Autodesk Inventor part; units mm, degrees
ref_plane "作業平面1" through (0, 0, 1.5) normal (0, 0, 1) x (1, 0, 0)
ref_plane "作業平面2" through (0, 0, 0.1) normal (0, 0, 1) x (1, 0, 0)
ref_plane "YZ Plane" through (0, 0, 0) normal (1, 0, 0) x (0, 1, 0)
sketch "スケッチ1" plane through (0, 0, 0) normal (0, 0, 1) x (1, 0, 0)
  line L0 (94.5, 10.9383) -> (94.5, -2.0617)
  line L1 (67.5, -2.0617) -> (67.5, -19.1729)
  line L2 (45.5, -19.1729) -> (45.5, -10.1729)
  line L3 (45.5, -10.1729) -> (63.5, -10.1729)
  line L4 (63.5, -10.1729) -> (63.5, -19.1729)
  line L5 (67.5, -19.1729) -> (63.5, -19.1729)
  line L6 (45.5, -19.1729) -> (41.5, -19.1729)
  line L7 (72.5, -2.0617) -> (72.5, 6.9383)
  line L8 (72.5, 6.9383) -> (90.5, 6.9383)
  line L9 (90.5, 6.9383) -> (90.5, -2.0617)
  line L10 (45.5, -19.1729) -> (55.5, -19.1729) construction
  line L11 (55.5, -19.1729) -> (55.5, -10.1729) construction
  line L12 (50.5, -19.1729) -> (50.5, 17.1682) construction
  line L13 (28.5, -2.0617) -> (28.5, 6.9383)
  line L14 (28.5, 6.9383) -> (10.5, 6.9383)
  line L15 (10.5, 6.9383) -> (10.5, -2.0617)
  line L16 (-17.5, 10.9383) -> (94.5, 10.9383)
  line L17 (94.5, -2.0617) -> (90.5, -2.0617)
  line L18 (72.5, -2.0617) -> (67.5, -2.0617)
  line L19 (6.5, -2.0617) -> (10.5, -2.0617)
  line L20 (6.5, -2.0617) -> (6.5, 6.9383)
  line L21 (6.5, 6.9383) -> (1.5, 6.9383)
  line L22 (72.5, -2.0617) -> (82.5, -2.0617) construction
  line L23 (82.5, -2.0617) -> (82.5, 6.9383) construction
  line L24 (77.5, -2.0617) -> (77.5, 30.8698) construction
  line L25 (28.5, -2.0617) -> (18.5, -2.0617) construction
  line L26 (18.5, -2.0617) -> (18.5, 6.9383) construction
  line L27 (23.5, -2.0617) -> (23.5, 26.9166) construction
  line L28 (41.5, -19.1729) -> (41.5, 6.9383)
  line L29 (41.5, 6.9383) -> (32.8043, 6.9383)
  line L30 (32.8043, 6.9383) -> (32.8043, -2.0617)
  line L31 (32.8043, -2.0617) -> (28.5, -2.0617)
  line L32 (68.5, 6.9383) -> (45.5, 6.9383)
  line L33 (45.5, 6.9383) -> (45.5, -6.1729)
  line L34 (45.5, -6.1729) -> (60.5869, -6.1729)
  line L35 (60.5869, -6.1729) -> (68.5, 1.7403)
  line L36 (68.5, 1.7403) -> (68.5, 6.9383)
  line L37 (0, -29.1814) -> (0, 40.8784)
  line L38 (1.5, 6.9383) -> (1.5, -8.0617)
  line L39 (1.5, -8.0617) -> (-17.5, -8.0617)
  line L40 (-17.5, -8.0617) -> (-17.5, 10.9383)
  circle A0 centre (-12.5, -2.0617) radius 2.25
  circle A1 centre (-3.5, -2.0617) radius 2.25
  line L41 (-12.5, -2.0617) -> (-3.5, -2.0617) construction
  point P0 (0, 0)
  point P1 (68.5, 4.3393)
  point P2 (68.5, 4.4383)
  dimension "d5" = 4
  dimension "d10" = 18
  dimension "d14" = 18
  dimension "d16" = 10
  dimension "d19" = 9
  dimension "d23" = 4
  dimension "d40" = 4
  dimension "d41" = 9
  dimension "d42" = 10
  dimension "d43" = 10
  dimension "d74" = 4
  dimension "d89" = 4
  dimension "d90" = 135
  dimension "d91" = 4
  dimension "d92" = 4
  dimension "d93" = 4
  dimension "d94" = 4
  dimension "d104" = 5
  dimension "d105" = 19
  dimension "d107" = 4.5
  dimension "d108" = 4.5
  dimension "d109" = 9
  dimension "d110" = 5
  dimension "d111" = 6
  dimension "d112" = 19
extrude "押し出し1" add sketch "スケッチ1" along normal mid plane 25 contours L0 L17 L9 L8 L7 L18 L1 L5 L4 L3 L2 L6 L28 L29 L30 L31 L13 L14 L15 L19 L20 L21 L38 L39 L37 L16 | L37 L39 L40 L16 | L36 L35 L34 L33 L32
sketch "スケッチ2" plane through (67.5, -19.1729, 12.5) normal (1, 0, 0) x (0, 0, -1)
  line L0 (6, 3) -> (19, 3)
  arc A0 (19, 3) -> (19, 7) centre (19, 5) ccw
  line L1 (19, 7) -> (6, 7)
  arc A1 (6, 7) -> (6, 3) centre (6, 5) ccw
  line L2 (25, 0) -> (0, 0)
  line L3 (25, 17.1112) -> (25, 0)
  line L4 (0, 0) -> (0, 17.1112)
  point P0 (12.5, 19.1729)
  point P1 (25, 13)
  point P2 (0, 13)
  dimension "d24" = 4
  dimension "d25" = 3
  dimension "d26" = 6
  dimension "d27" = 6
extrude "押し出し2" cut sketch "スケッチ2" against normal up to surface (4 mm away)
chamfer "面取り1" distance 2 angle 45 1 edges at (63.5, -10.1729, 0)
sketch "スケッチ4" plane through (94.5, -2.0617, 12.5) normal (1, 0, 0) x (0, 0, -1)
  line L0 (6, 3) -> (19, 3)
  arc A0 (19, 3) -> (19, 7) centre (19, 5) ccw
  line L1 (19, 7) -> (6, 7)
  arc A1 (6, 7) -> (6, 3) centre (6, 5) ccw
  line L2 (25, 13) -> (25, 0)
  line L3 (0, 0) -> (0, 13)
  line L4 (25, 0) -> (0, 0)
  point P0 (12.5, 2.0617)
  dimension "d45" = 4
  dimension "d46" = 6
  dimension "d47" = 6
  dimension "d48" = 3
extrude "押し出し3" cut sketch "スケッチ4" against normal up to surface (4 mm away)
sketch "スケッチ5" plane through (6.5, -2.0617, 12.5) normal (-1, 0, 0) x (0, 0, 1)
  line L0 (-19, 3) -> (-6, 3)
  line L1 (-19, 3) -> (-6, 3)
  arc A0 (-6, 3) -> (-6, 7) centre (-6, 5) ccw
  line L2 (-6, 7) -> (-19, 7)
  line L3 (-6, 7) -> (-19, 7)
  arc A1 (-19, 7) -> (-19, 3) centre (-19, 5) ccw
  point P0 (-12.5, 2.0617)
  point P1 (-6, 7)
extrude "押し出し4" cut sketch "スケッチ5" against normal up to surface (4 mm away)
chamfer "面取り4" distance 2 angle 45 3 edges at (90.5, 6.9383, 0) (10.5, 6.9383, 0) (6.5, 6.9383, 0)
ref_plane "作業平面1" through (0, 0, 1.5) normal (0, 0, 1) x (1, 0, 0)
ref_plane "作業平面2" through (0, 0, 0.1) normal (0, 0, 1) x (1, 0, 0)
properties part number "adapter_ver.1"
Source: CAD feature listing. Evaluate the final solid. Frame: model axes, mm. A direction names the side the tool comes from. Coordinates: 2 decimals unless noted, no trailing zeros. Loops run counter-clockwise (first coordinate to the right, second up) from the corner with the lowest first, then second, coordinate; pieces in that order, holes last. Notation, with made-up numbers: (11.5, 13.5) - (65.5, 13.5) arc R22 ccw to (65.5, 29.5) - close; hole circle Ø1 at (15, 30.5). An arc over 180 degrees is marked (long way). One line per item, written item: value. Start each with the question number.
1. Section C-C (y = 2). Return the cut outline in (x, z), and give its area (3 significant figures).
2. Mould query, pull axis Z, two halves, no side actions, for faces 6 (the cylindrical face through (8.5, 2.9, 8.5)), 7 (the flat face through (63.5, -16.4, -0.2)), 8 (the flat face through (42, 0, -12.5)). Classes: pulls with the +Z half, pulls with the -Z half, needs draft (parallel to the pull), parting line crosses it, or undercut.
3. Set-up query: faces 1 (the flat face through (28.5, 2, 0)), 2 (the flat face through (93, 0.938, 0)), 3 (the flat face through (93, -2.062, 0)), 4 (the flat face through (-17.5, 1, 0)), 5 (the flat face through (8, 4.938, 0)). Return all of +Z, -Z, +X, -X, +Y, -Y with unobstructed straight access to the full face (end or side cutting, diameter ignored); none if empty.
4. Ray query, L1, parallel to X at y = 4, z = -10.5; L2, parallel to X at y = 4.5, z = 5; L3, parallel to X at y = -5.5, z = -6.5. Return the intervals inside material, ascending.
5. Contact query for flat-ended pins moving along their axis: P1, Ø10, axis at y = -15.5, z = 1.5, coming from the +X side; P2, Ø5, axis at x = 84, z = -0.5, coming from the -Y side; P3, Ø4.5, axis at x = 93, z = 0, coming from the -Y side; P4, Ø2, axis at x = 11, y = 3, coming from the +Z side. Output: stop coordinate, or through.
6. Section B-B (x = -3.5). Return the cut outline in (y, z), and give its area (4 significant figures).
7. Section A-A (z = -9.5). State how many separate pieces and enclosed holes the cut face has, and give its area (3 significant figures).
Verdict:
1. outline: (-17.5, -12.5) - (1.5, -12.5) - (1.5, 12.5) - (-17.5, 12.5) - close; (6.5, -12.5) - (10.5, -12.5) - (10.5, -8.27) - (6.5, -8.27) - close; (6.5, 8.27) - (10.5, 8.27) - (10.5, 12.5) - (6.5, 12.5) - close; (28.5, -12.5) - (32.8, -12.5) - (32.8, 12.5) - (28.5, 12.5) - close; (41.5, -12.5) - (72.5, -12.5) - (72.5, 12.5) - (41.5, 12.5) - close; (90.5, -12.5) - (94.5, -12.5) - (94.5, -8.27) - (90.5, -8.27) - close; (90.5, 8.27) - (94.5, 8.27) - (94.5, 12.5) - (90.5, 12.5) - close
1. area: 1,430 mm2
2. face 6: undercut
2. face 7: needs draft
2. face 8: pulls with the -Z half
3. face 1: +Z, -Z, -Y
3. face 2: +X
3. face 3: +Z, -Z, +X, -Y
3. face 4: +Z, -Z, -X, +Y, -Y
3. face 5: none
4. L1: x = -17.5 to 1.5, 6.5 to 10.5, 28.5 to 32.8, 41.5 to 72.5, 90.5 to 94.5
4. L2: x = -17.5 to 1.5, 28.5 to 32.8, 41.5 to 72.5
4. L3: x = -17.5 to 1.5, 41.5 to 67.5
5. P1: stops at x = 67.5
5. P2: stops at y = 6.94
5. P3: stops at y = -2.06
5. P4: stops at z = 12.5
6. outline: (-8.06, -12.5) - (-4.31, -12.5) - (-4.31, 12.5) - (-8.06, 12.5) - close; (0.19, -12.5) - (10.94, -12.5) - (10.94, 12.5) - (0.19, 12.5) - close
6. area: 362.5 mm2
7. separate pieces: 1
7. enclosed holes: 2
7. area: 1,380 mm2
